Build history of the part. All positions in model axes, mm. A direction names the side the tool comes from. Round coordinates to 2 decimals unless told otherwise and drop trailing zeros. Order: outer loops, then holes, each group sorted by start corner. A loop starts at its lowest first (then second) coordinate and runs counter-clockwise, first axis right, second up. Notation, with made-up numbers: (-35, 1.25) -> (11, 1.25) arc R23 cw to (11, 14.25) -> close; hole circle Ø4 at (84, 15.25). An arc over 180 degrees is marked (long way). Answer as CSV lines item,"result". Start each with the question number.
```python
from build123d import *

# Parameters (mm, degrees)
F1_DEPTH = 30
F3_DEPTH = 25
F4_W     = 8
F4_H     = 10
F4_W_2   = 12
F5_DEPTH = 1
F7_D     = 3.3


with BuildPart() as f1:
    # F0 (on Top) → F1 (new body)
    with BuildSketch(Plane.XY):
        Polygon((-115, 0), (-115, -1), (-105, -1), (-105, 9), (105, 9), (105, 0), (115, 0), (115, 1), (106, 1), (106, 10), (-106, 10), (-106, 0), align=None)
    extrude(amount=F1_DEPTH)

    # F2 (on face) → F3 (cut)
    with BuildSketch(Plane(origin=(0, 1, 0), x_dir=(-1, 0, 0), z_dir=(0, 1, 0))):
        with BuildLine():
            Line((-109.25, 5), (-109.25, 25))
            ThreePointArc((-109.25, 25), (-111, 26.75), (-112.75, 25))
            Line((-112.75, 25), (-112.75, 5))
            ThreePointArc((-112.75, 5), (-111, 3.25), (-109.25, 5))
        make_face()
        with BuildLine():
            Line((109.25, 25), (109.25, 5))
            ThreePointArc((109.25, 5), (111, 3.25), (112.75, 5))
            Line((112.75, 5), (112.75, 25))
            ThreePointArc((112.75, 25), (111, 26.75), (109.25, 25))
        make_face()
    extrude(amount=-F3_DEPTH, mode=Mode.SUBTRACT)

    # F4 (on face) → F5 (join)
    with BuildSketch(Plane.XZ.offset(-9)):
        with Locations((-101, -5)):
            Rectangle(F4_W, F4_H)
        with Locations((-92, -5)):
            Rectangle(F4_W, F4_H)
        with Locations((-83, -5)):
            Rectangle(F4_W, F4_H)
        with Locations((-74, -5)):
            Rectangle(F4_W, F4_H)
        with Locations((-65, -5)):
            Rectangle(F4_W, F4_H)
        with Locations((-56, -5)):
            Rectangle(F4_W, F4_H)
        with Locations((-47, -5)):
            Rectangle(F4_W, F4_H)
        with Locations((-38, -5)):
            Rectangle(F4_W, F4_H)
        with Locations((-29, -5)):
            Rectangle(F4_W, F4_H)
        with Locations((-20, -5)):
            Rectangle(F4_W, F4_H)
        with Locations((-11, -5)):
            Rectangle(F4_W, F4_H)
        with Locations((101, -5)):
            Rectangle(F4_W, F4_H)
        with Locations((92, -5)):
            Rectangle(F4_W, F4_H)
        with Locations((83, -5)):
            Rectangle(F4_W, F4_H)
        with Locations((74, -5)):
            Rectangle(F4_W, F4_H)
        with Locations((65, -5)):
            Rectangle(F4_W, F4_H)
        with Locations((56, -5)):
            Rectangle(F4_W, F4_H)
        with Locations((47, -5)):
            Rectangle(F4_W, F4_H)
        with Locations((38, -5)):
            Rectangle(F4_W, F4_H)
        with Locations((29, -5)):
            Rectangle(F4_W, F4_H)
        with Locations((20, -5)):
            Rectangle(F4_W, F4_H)
        with Locations((11, -5)):
            Rectangle(F4_W, F4_H)
        with Locations((0, -5)):
            Rectangle(F4_W_2, F4_H)
    extrude(amount=-F5_DEPTH)

    # F7 (through all)
    with Locations(Plane(origin=(0, 10, 0), x_dir=(-1, 0, 0), z_dir=(0, 1, 0))):
        with Locations((0, 15), (0, 25)):
            Hole(F7_D / 2)


solid = f1.part
```
Q1. Two-plate mould, pull along X, no slides. Class faces 6 (the face through (105, 5, 15)), 7 (the face through (106, 5, 15)), 8 (the face through (-105, 4, 15)), 9 (the face through (-1, 10, 10)): +X half, -X half, draft (parallel to the pull), parting line (faces both ways), or undercut.
Q2. Slice it at A-A, the plane y = 4.5. Write the cut outline in (x, z), plus the area to 3 significant figures.
Q3. Slice it at C-C, the plane x = -22. Write the cut outline in (y, z).
Q4. Flat gauge pins, fed straight in: pin 1 Ø0.8 at (y, z) = (9.5, -7) entering from -X; pin 2 Ø0.8 at (y, z) = (9.5, -5.5) entering from +X; pin 3 Ø1.5 at (x, z) = (-88.5, 13.5) entering from -Y; pin 4 Ø5 at (x, y) = (69, 5) entering from +Z. Where does each tip first touch, or does it go through?
Q5. Probe L1, parallel to Z at x = 0, y = 9.4; L2, parallel to X at y = 2.75, z = 20; L3, parallel to Y at x = -103.5, z = 3. List the from-to ranges inside material, lowest first.
Q6. Which spindle directions (+Z, -Z, +X, -X, +Y, -Y) get a long thin tool onto all of the face, cutting with end or side? Do faces 1 (the face through (-106, 5, 15)), 2 (the face through (109, 0, 15)), 3 (the face through (109, 1, 15)), 4 (the face through (-109, -1, 15)), 5 (the face through (-1, 9, 10)). Say none if no direction does.
Q7. Slice it at B-B, the plane z = 21. Write the cut outline in (x, y).
Solutions:
1,face 6,"undercut"
1,face 7,"+X half"
1,face 8,"undercut"
1,face 9,"draft"
2,outline,"(-106, 0) -> (-105, 0) -> (-105, 30) -> (-106, 30) -> close; (105, 0) -> (106, 0) -> (106, 30) -> (105, 30) -> close"
2,area,"60.0 mm2"
3,outline,"(9, -10) -> (10, -10) -> (10, 30) -> (9, 30) -> close"
4,pin 1,"stops at x = -105"
4,pin 2,"stops at x = 105"
4,pin 3,"stops at y = 9"
4,pin 4,"passes through"
5,L1,"z = -10 to 13.35, 16.65 to 23.35, 26.65 to 30"
5,L2,"x = -106 to -105, 105 to 106"
5,L3,"y = 9 to 10"
6,face 1,"+Z, -Z, -X, +Y"
6,face 2,"+Z, -Z, +X, -Y"
6,face 3,"+Z, -Z, +X, +Y"
6,face 4,"+Z, -Z, +X, -X, -Y"
6,face 5,"+Z, -Z, -Y"
7,outline,"(-115, -1) -> (-112.75, -1) -> (-112.75, 0) -> (-115, 0) -> close; (-109.25, -1) -> (-105, -1) -> (-105, 9) -> (105, 9) -> (105, 0) -> (109.25, 0) -> (109.25, 1) -> (106, 1) -> (106, 10) -> (-106, 10) -> (-106, 0) -> (-109.25, 0) -> close; (112.75, 0) -> (115, 0) -> (115, 1) -> (112.75, 1) -> close"
